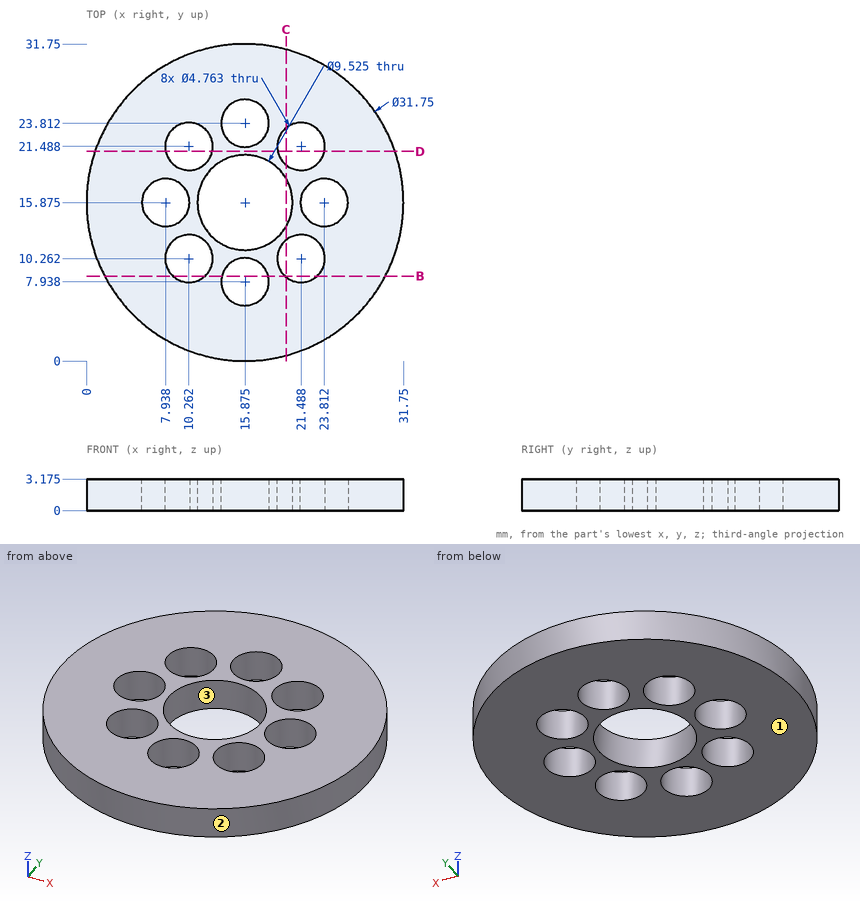
Study the drawing (mm; zero at the part's minimum x, y, z) and answer. Round coordinates to 2 decimals unless told otherwise and drop trailing zeros. Write each loop counter-clockwise with the first axis right and the second up, starting at its lowest first coordinate (ties: lowest second). Pieces come first, ordered by that corner, then holes. Notation, with made-up numbers: (23.25, 43.5) - (57.25, 43.5) arc R25 ccw to (57.25, 78.5) - close; hole circle Ø8 at (86, 0). An arc over 180 degrees is marked (long way). Return JSON: item names as keys, results as strings. Group by question number.
Q1. The part is cut by section D-D on y = 21. Count the separate pieces of the cut face and the enclosed holes in it.
Q2. The part is cut by section B-B on y = 8.5. Write down the section's boundary in (x, z) (1 decimal).
Q3. The part is cut by section C-C on x = 20. Write down the section's boundary in (y, z) (1 decimal).
Q4. Each of these flat-tipped pins is pushed along its axis until it touches: pin 1 Ø1.5 at (x, z) = (10.5, 1) entering from -Y; pin 2 Ø1.5 at (x, z) = (28.5, 1) entering from -Y; pin 3 Ø1 at (x, z) = (20, 0.5) entering from -Y; pin 4 Ø4.5 at (x, y) = (7.94, 15.88) entering from -Z. Where does it stop, or does it pass through?
Q5. Find the intervals of material crossed by L1, parallel to X at y = 15, z = 0.8 (1 decimal); L2, parallel to Y at x = 14.5, z = 1.6 (1 decimal); L3, parallel to X at y = 12, z = 1.1 (1 decimal), in increasing order.
Q6. The mould has two halves that part along Y. Classify the marked faces 1, 2 and 3: released by +Y, released by -Y, zero draft, split by the parting line, or undercut.
Solved:
{
 "1": {"separate pieces": "3", "enclosed holes": "0"},
 "2": {"outline": "(1.8, 0) - (8.7, 0) - (8.7, 3.2) - (1.8, 3.2) - close; (11.9, 0) - (13.6, 0) - (13.6, 3.2) - (11.9, 3.2) - close; (18.2, 0) - (19.9, 0) - (19.9, 3.2) - (18.2, 3.2) - close; (23.1, 0) - (29.9, 0) - (29.9, 3.2) - (23.1, 3.2) - close"},
 "3": {"outline": "(0.5, 0) - (8.4, 0) - (8.4, 3.2) - (0.5, 3.2) - close; (12.1, 0) - (13.5, 0) - (13.5, 3.2) - (12.1, 3.2) - close; (18.3, 0) - (19.6, 0) - (19.6, 3.2) - (18.3, 3.2) - close; (23.3, 0) - (31.2, 0) - (31.2, 3.2) - (23.3, 3.2) - close"},
 "4": {"pin 1": "y = 0.69", "pin 2": "y = 5.34", "pin 3": "y = 0.42", "pin 4": "through"},
 "5": {"L1": "0 to 5.7, 10.2 to 11.2, 20.6 to 21.6, 26 to 31.7", "L2": "0.1 to 6, 9.9 to 11.3, 20.4 to 21.9, 25.8 to 31.7", "L3": "0.5 to 8.6, 11.9 to 13.1, 18.6 to 19.9, 23.1 to 31.3"},
 "6": {"face 1": "zero draft", "face 2": "split by the parting line", "face 3": "undercut"}
}
